Geometry check sheet. Reference: the model listing, model coordinates, mm. A direction names the side the tool comes from. Coordinates: 2 decimals unless noted, no trailing zeros. Write each loop counter-clockwise with the first axis right and the second up, starting at its lowest first coordinate (ties: lowest second). Pieces come first, ordered by that corner, then holes. Notation, with made-up numbers: M 78,33 L 89,33 A25 cw 89,54 Z; hole C 86,-30 d3. An arc over 180 degrees is marked long. Answer as a JSON object with one key per item and string values. Group by question number.
```python
from build123d import *

# Parameters (mm, degrees)
SKETCH2_W           = 26
SKETCH2_H           = 30
BOSS_EXTRUDE1_DEPTH = 93.4
SKETCH3_R           = 9.2
CUT_EXTRUDE1_DEPTH  = 8
CUT_EXTRUDE2_START  = -8
SKETCH4_R           = 9.2
CUT_EXTRUDE2_DEPTH  = 8
FILLET1_R           = 15
FILLET4_R           = 10
FILLET5_R           = 10


# Some blends are built 0.0001 mm under size
with BuildPart() as part:
    # Sketch2 → Boss-Extrude1 (new body)
    with BuildSketch(Plane(origin=(0, 0, 0), x_dir=(1, 0, 0), z_dir=(0, 1, 0))):
        Rectangle(SKETCH2_W, SKETCH2_H)
    extrude(amount=BOSS_EXTRUDE1_DEPTH)

    # Sketch3 → Cut-Extrude1 (cut)
    with BuildSketch(Plane(origin=(13, 0, 0), x_dir=(0, 0, -1), z_dir=(1, 0, 0))):
        with Locations((0, 69)):
            Circle(SKETCH3_R)
    extrude(amount=-CUT_EXTRUDE1_DEPTH, mode=Mode.SUBTRACT)

    # Sketch4 → Cut-Extrude2 (cut)
    with BuildSketch(Plane.ZY.offset(13).offset(CUT_EXTRUDE2_START)):
        with Locations(Location((0, 69, 0), (0, 0, 180))):
            Circle(SKETCH4_R)
    extrude(amount=CUT_EXTRUDE2_DEPTH, mode=Mode.SUBTRACT)

    # Fillet1
    fillet1_edges = [part.edges().sort_by_distance(p)[0] for p in [
        (0, 93.4, 15),
        (0, 93.4, -15),
    ]]
    fillet(fillet1_edges, radius=FILLET1_R - 0.0001)  # a hair under: the kernel refuses the full size

    # Fillet4
    # the kernel refuses this fillet: 10 mm, written as the material it takes off along each edge
    with BuildSketch(Plane(origin=(-13, -25, 15), x_dir=(0, 0, -1), z_dir=(0, 1, 0)), Plane(origin=(-13, -25, -15), x_dir=(1, 0, 0), z_dir=(0, 1, 0))) as fillet4_piece_1:
        with BuildLine():
            CenterArc((FILLET4_R, -FILLET4_R), FILLET4_R, 90, 90)
            Line((0, -FILLET4_R), (0, 0))
            Line((0, 0), (FILLET4_R, 0))
        make_face()
    extrude(amount=103.4001, mode=Mode.SUBTRACT)
    with BuildSketch(Plane(origin=(-13, 78.4001, -0.0001), x_dir=(0, 0, -1), z_dir=(0, -1, 0))) as fillet4_piece_2:
        with BuildLine():
            CenterArc((14.9999 - FILLET4_R, FILLET4_R), FILLET4_R, 270, 90)
            Line((14.9999, FILLET4_R), (14.9999, 0))
            Line((14.9999, 0), (14.9999 - FILLET4_R, 0))
        make_face()
    revolve(axis=Axis((-13, 78.4001, -0.0001), (1, 0, 0)), revolution_arc=90, mode=Mode.SUBTRACT)
    with BuildSketch(Plane(origin=(-13, 78.4001, 0.0001), x_dir=(0, 1, 0), z_dir=(0, 0, -1))) as fillet4_piece_3:
        with BuildLine():
            CenterArc((14.9999 - FILLET4_R, FILLET4_R), FILLET4_R, 270, 90)
            Line((14.9999, FILLET4_R), (14.9999, 0))
            Line((14.9999, 0), (14.9999 - FILLET4_R, 0))
        make_face()
    revolve(axis=Axis((-13, 78.4001, 0.0001), (1, 0, 0)), revolution_arc=90, mode=Mode.SUBTRACT)
    with BuildSketch(Plane(origin=(-13, 93.4, 0.0001), x_dir=(0, -1, 0), z_dir=(0, 0, -1))) as fillet4_piece_4:
        with BuildLine():
            CenterArc((FILLET4_R, -FILLET4_R), FILLET4_R, 90, 90)
            Line((0, -FILLET4_R), (0, 0))
            Line((0, 0), (FILLET4_R, 0))
        make_face()
    extrude(amount=0.0002, mode=Mode.SUBTRACT)

    # Fillet5
    # the kernel refuses this fillet: 10 mm, written as the material it takes off along each edge
    with BuildSketch(Plane(origin=(13, -25, -15), x_dir=(-1, 0, 0), z_dir=(0, 1, 0)), Plane(origin=(13, -25, 15), x_dir=(0, 0, -1), z_dir=(0, 1, 0))) as fillet5_piece_1:
        with BuildLine():
            CenterArc((FILLET5_R, FILLET5_R), FILLET5_R, 180, 90)
            Line((0, FILLET5_R), (0, 0))
            Line((0, 0), (FILLET5_R, 0))
        make_face()
    extrude(amount=103.4001, mode=Mode.SUBTRACT)
    with BuildSketch(Plane(origin=(13, 78.4001, -0.0001), x_dir=(0, 0, -1), z_dir=(0, -1, 0))) as fillet5_piece_2:
        with BuildLine():
            CenterArc((14.9999 - FILLET5_R, -FILLET5_R), FILLET5_R, 0, 90)
            Line((14.9999, -FILLET5_R), (14.9999, 0))
            Line((14.9999, 0), (14.9999 - FILLET5_R, 0))
        make_face()
    revolve(axis=Axis((13, 78.4001, -0.0001), (1, 0, 0)), revolution_arc=90, mode=Mode.SUBTRACT)
    with BuildSketch(Plane(origin=(13, 78.4001, 0.0001), x_dir=(0, 1, 0), z_dir=(0, 0, -1))) as fillet5_piece_3:
        with BuildLine():
            CenterArc((14.9999 - FILLET5_R, -FILLET5_R), FILLET5_R, 0, 90)
            Line((14.9999, -FILLET5_R), (14.9999, 0))
            Line((14.9999, 0), (14.9999 - FILLET5_R, 0))
        make_face()
    revolve(axis=Axis((13, 78.4001, 0.0001), (1, 0, 0)), revolution_arc=90, mode=Mode.SUBTRACT)
    with BuildSketch(Plane(origin=(13, 93.4, -0.0001), x_dir=(0, -1, 0), z_dir=(0, 0, 1))) as fillet5_piece_4:
        with BuildLine():
            CenterArc((FILLET5_R, -FILLET5_R), FILLET5_R, 90, 90)
            Line((0, -FILLET5_R), (0, 0))
            Line((0, 0), (FILLET5_R, 0))
        make_face()
    extrude(amount=0.0002, mode=Mode.SUBTRACT)


solid = part.part
```
1) Draft check along Y on faces 1 (the cylindrical face through (0.04, 88.89, 10.72)), 2 (the flat face through (0, 0, 0)), 3 (the flat face through (5, 69, 0)). Enter one of: +Y half, -Y half, draft (parallel to the pull), parting line (faces both ways), or undercut.
2) Section check C-C (y = 69). Record the cut outline in (x, z), then the cut area to 3 significant figures.
3) Set-up check for faces 4 (the flat face through (-5, 69, 0)), 5 (the cylindrical face through (9.06, 69.4, 9.19)), 6 (the cylindrical face through (-9.99, 38.65, -12.15)): record each of +Z, -Z, +X, -X, +Y, -Y from which the full face is reachable in a straight line by a thin tool's end or side.
4) Section check A-A (y = 36). Record the cut outline in (x, z).
5) Material ranges on probe 1 along Y at (x, z) = (6, 2); probe 2 along Z at (x, y) = (-9.75, 69); probe 3 along Y at (x, z) = (7.25, 0), recorded low to high. Write a range as [from, to].
6) Go/stop test with flat-tipped pins: pin 1 Ø8 at (x, z) = (2.5, 5.5) entering from +Y; pin 2 Ø5 at (x, z) = (4, -5.5) entering from +Y; pin 3 Ø1 at (x, y) = (4, 61.5) entering from -Z. Record where each tip stops, or that it passes through.
Entries:
{
 "1": {"face 1": "+Y half", "face 2": "-Y half", "face 3": "undercut"},
 "2": {"outline": "M -12.08,-9.2 A10 ccw -3,-15 L 3,-15 A10 ccw 12.08,-9.2 L 5,-9.2 L 5,9.2 L 12.08,9.2 A10 ccw 3,15 L -3,15 A10 ccw -12.08,9.2 L -5,9.2 L -5,-9.2 Z", "area": "405 mm^2"},
 "3": {"face 4": "-X", "face 5": "+X", "face 6": "-Z, -X, +Y, -Y"},
 "4": {"outline": "M -13,-5 A10 ccw -3,-15 L 3,-15 A10 ccw 13,-5 L 13,5 A10 ccw 3,15 L -3,15 A10 ccw -13,5 Z"},
 "5": {"probe 1": "[0, 60.02], [77.98, 92.8]", "probe 2": "[-12.38, -9.2], [9.2, 12.38]", "probe 3": "[0, 59.8], [78.2, 92.45]"},
 "6": {"pin 1": "y = 93.32", "pin 2": "y = 93.07", "pin 3": "z = -14.99"}
}
